from build123d import *

# Parameters (mm, degrees)
F0_W      = 63.641474
F0_H      = 41.773599
F0_W_2    = 49.73047
F0_H_2    = 29.838283
F1_DEPTH  = 57.15
F2_R      = 19.05
F2_R_2    = 6.35
F2_R_3    = 31.75
F2_R_4    = 12.7
F3_DEPTH  = 25.4
F4_R      = 31.75
F4_R_2    = 12.7
F4_R_3    = 19.05
F4_R_4    = 6.35
F5_DEPTH  = 25.4
F6_W      = 40.11992
F6_H      = 29.025927
F7_DEPTH  = 25.4
F8_R      = 5.08
F9_W      = 16.103194
F9_H      = 9.219451
F9_W_2    = 7.053554
F9_H_2    = 3.602702
F10_DEPTH = 20.32
F11_W     = 57.042776
F11_H     = 9.006755
F11_W_2   = 6.004483
F11_H_2   = 24.91869
F11_W_3   = 5.704254
F11_H_3   = 23.417564
F11_H_4   = 24.618464
F11_W_4   = 6.004482
F11_H_5   = 23.717788
F12_DEPTH = 63.246


with BuildPart() as f1:
    # F0 (on Front) → F1 (new body)
    with BuildSketch(Plane.XZ):
        Polygon((-63.641474, 24.699468), (-63.655011, 24.699468), (-63.655011, -27.683297), (70.948809, -27.683297), (70.948809, 24.699468), (0, 24.699468), align=None)
        with Locations((-31.820737, 45.586267)):
            Rectangle(F0_W, F0_H)
        with Locations((-33.816721, 45.586267)):
            Rectangle(F0_W_2, F0_H_2, mode=Mode.SUBTRACT)
    extrude(amount=F1_DEPTH)

    # F2 (on Front) → F3 (join)
    with BuildSketch(Plane.XZ):
        with Locations((47.813714, -36.03467)):
            Circle(F2_R)
        with Locations((47.813714, -36.03467)):
            Circle(F2_R_2, mode=Mode.SUBTRACT)
        with Locations((-38.951659, -27.168135)):
            Circle(F2_R_3)
        with Locations((-38.951659, -27.168135)):
            Circle(F2_R_4, mode=Mode.SUBTRACT)
    extrude(amount=-F3_DEPTH)

    # F4 (on face) → F5 (join)
    with BuildSketch(Plane.XZ.offset(57.15)):
        with Locations((-38.965259, -27.683297)):
            Circle(F4_R)
        with Locations((-38.965259, -27.683297)):
            Circle(F4_R_2, mode=Mode.SUBTRACT)
        with Locations((47.799807, -36.177129)):
            Circle(F4_R_3)
        with Locations((47.799807, -36.177129)):
            Circle(F4_R_4, mode=Mode.SUBTRACT)
    extrude(amount=F5_DEPTH)

    # F6 (on face) → F7 (cut)
    with BuildSketch(Plane.YZ):
        with Locations((-28.575, 45.586267)):
            Rectangle(F6_W, F6_H)
    extrude(amount=-F7_DEPTH, mode=Mode.SUBTRACT)

    # F8
    f8_edges = [f1.edges().sort_by_distance(p)[0] for p in [
        (0, -28.575, 24.699468),
        (70.948809, -28.575, 24.699468),
        (70.948809, -28.575, -27.683297),
        (70.948809, 0, -1.491915),
        (70.948809, -57.15, -1.491915),
        (-31.820737, -57.15, 66.473067),
        (0, -28.575, 66.473067),
        (-31.820737, 0, 66.473067),
        (-63.641474, -28.575, 66.473067),
    ]]
    fillet(f8_edges, radius=F8_R)

    # F9 (on face) → F10 (join)
    with BuildSketch(Plane(origin=(-63.655011, 0, 0), x_dir=(0, -1, 0), z_dir=(-1, 0, 0))):
        with Locations((45.752488, -23.073571)):
            Rectangle(F9_W, F9_H)
        with Locations((45.752488, -23.074446)):
            Rectangle(F9_W_2, F9_H_2, mode=Mode.SUBTRACT)
    extrude(amount=F10_DEPTH)

    # F11 (on face) → F12 (cut)
    with BuildSketch(Plane.XZ.offset(57.15)):
        with Locations((37.286255, 17.56317)):
            Rectangle(F11_W, F11_H)
        with Locations((15.67004, -2.852139)):
            Rectangle(F11_W_2, F11_H_2)
        with Locations((26.778372, -2.852139)):
            Rectangle(F11_W_3, F11_H_3)
        with Locations((46.293005, -2.852139)):
            Rectangle(F11_W_2, F11_H_4)
        with Locations((37.286252, -2.852139)):
            Rectangle(F11_W_4, F11_H_5)
    extrude(amount=-F12_DEPTH, mode=Mode.SUBTRACT)


solid = f1.part
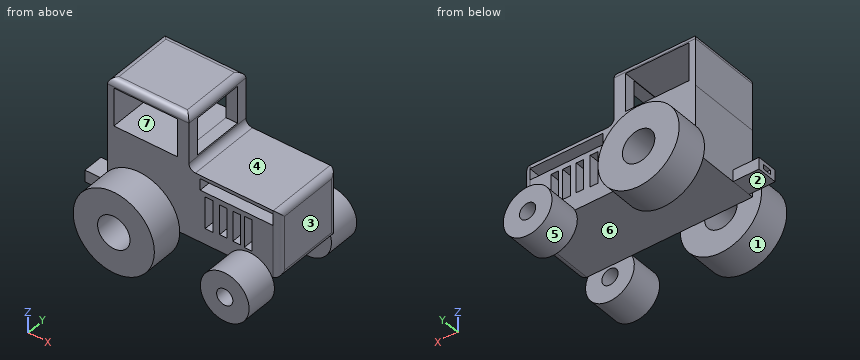
Model file for the job. Use its own axes, mm. Face numbers are marked on the shaded views. A direction names the side the tool comes from. Round coordinates to 2 decimals unless told otherwise and drop trailing zeros. Loops run counter-clockwise (first coordinate to the right, second up) from the corner with the lowest first, then second, coordinate; pieces in that order, holes last.
1. Tool access for the marked faces 4, 5, 6 and 7: list every direction of +Z, -Z, +X, -X, +Y, -Y with a clear straight run to the whole face (end or side of a thin tool).
Check values:
face 4: +Z, +X, +Y, -Y
face 5: +Y
face 6: -Z, +X, -X
face 7: +Y, -Y
2. Drop flat-ended pins along their axis: P1, Ø6, axis at x = -24, y = 0, coming from the +Z side; P2, Ø7, axis at x = -3.5, z = 47, coming from the -Y side; P3, Ø4, axis at y = -53.5, z = 31.5, coming from the -X side; P4, Ø11.5, axis at x = 47.81, z = -36.03, coming from the +Y side. Give the stop position or say it passes through.
Check values:
P1: stops at z = 66.03
P2: stops at y = -57.15
P3: stops at x = -63.64
P4: passes through
3. Band-saw the part on B-B, the plane x = -31.5. List the corners of the cut face in (y, z).
Check values:
outline: (-82.55, -58.54) - (-57.15, -58.54) - (-57.15, -37.96) - (-82.55, -37.96) - close; (-82.55, -17.41) - (-57.15, -17.41) - (-57.15, -27.68) - (0, -27.68) - (0, -16.88) - (25.4, -16.88) - (25.4, 3.7) - (0, 3.7) - (0, 30.67) - (-57.15, 30.67) - (-57.15, 3.18) - (-82.55, 3.18) - close; (-57.15, 60.51) - (0, 60.51) - (0, 61.39) arc R5.08 ccw to (-5.08, 66.47) - (-52.07, 66.47) arc R5.08 ccw to (-57.15, 61.39) - close; (0, -58.03) - (25.4, -58.03) - (25.4, -37.45) - (0, -37.45) - close
4. Band-saw the part on D-D, the plane x = -67.5. List the corners of the cut face in (y, z).
Check values:
outline: (-82.55, -41.61) - (-57.15, -41.61) - (-57.15, -13.76) - (-82.55, -13.76) - close; (-53.8, -27.68) - (-37.7, -27.68) - (-37.7, -18.46) - (-53.8, -18.46) - close; (0, -41.06) - (25.4, -41.06) - (25.4, -13.27) - (0, -13.27) - close; hole (-49.28, -24.88) - (-42.23, -24.88) - (-42.23, -21.27) - (-49.28, -21.27) - close
5. Mould opens along X. For the marked faces 1, 2 and 3 say: +X half, -X half, draft (parallel to the pull), parting line (faces both ways), or undercut.
Check values:
face 1: undercut
face 2: draft
face 3: +X half
6. Band-saw the part on A-A, the plane z = 44. List the corners of the cut face in (x, y), and give its area (3 significant figures).
Check values:
outline: (-63.64, -57.15) - (-58.68, -57.15) - (-58.68, 0) - (-63.64, 0) - close; (-8.95, -57.15) - (0, -57.15) - (0, -48.63) - (-8.95, -48.63) - close; (-8.95, -8.52) - (0, -8.52) - (0, 0) - (-8.95, 0) - close
area: 436 mm2
7. Wall check: probe 1 along X at (y, z) = (-31.5, -8.5); probe 2 along Y at (x, z) = (-13, -37); probe 3 along Z at (x, y) = (12, -21). Give the ranges that are in metal, low to high.
Check values:
probe 1: x = -63.66 to 12.67, 18.67 to 23.93, 29.63 to 34.28, 40.29 to 43.29, 49.3 to 70.95
probe 2: y = -82.55 to -57.15, 0 to 25.4
probe 3: z = -27.68 to 13.06, 22.07 to 24.7
8. Band-saw the part on C-C, the plane z = 15. List the corners of the cut face in (x, y), and give its area (3 significant figures).
Check values:
outline: (-63.66, -57.15) - (8.76, -57.15) - (8.76, 0) - (-63.66, 0) - close; (65.81, -57.15) - (65.87, -57.15) arc R5.08 ccw to (70.95, -52.07) - (70.95, -5.08) arc R5.08 ccw to (65.87, 0) - (65.81, 0) - close
area: 4,420 mm2
